```python
from build123d import *

# Parameters (mm, degrees)
F0_W     = 508
F0_H     = 457.2
F0_W_2   = 152.4
F0_H_2   = 101.6
F1_DEPTH = 12.7
F2_W     = 508
F2_H     = 228.6
F3_DEPTH = 12.701
F5_DEPTH = 12.701
F7_DEPTH = 9.525


with BuildPart() as f1:
    # F0 (on Top) → F1 (new body)
    with BuildSketch(Plane.XY):
        with Locations((76.2, -50.8)):
            Rectangle(F0_W, F0_H)
        with Locations((76.2, -50.8)):
            Rectangle(F0_W_2, F0_H_2, mode=Mode.SUBTRACT)
    extrude(amount=F1_DEPTH)

    # F2 (on face) → F3 (cut, through all)
    with BuildSketch(Plane.XY.offset(12.7)):
        with Locations((76.2, 63.5)):
            Rectangle(F2_W, F2_H)
    extrude(amount=-F3_DEPTH, mode=Mode.SUBTRACT)

    # F4 (on face) → F5 (cut, through all)
    with BuildSketch(Plane.XY.offset(12.7)):
        Polygon((-12.7, -63.5), (-165.1, -63.5), (-165.1, -266.7), (317.5, -266.7), (317.5, -63.5), (165.1, -63.5), (165.1, -114.3), (-12.7, -114.3), align=None)
    extrude(amount=-F5_DEPTH, mode=Mode.SUBTRACT)

    # F6 (on face) → F7 (cut)
    with BuildSketch(Plane(origin=(0, 0, 0), x_dir=(1, 0, 0), z_dir=(0, 0, -1))):
        Polygon((-174.625, 276.225), (-174.625, 53.975), (-3.175, 53.975), (-3.175, 104.775), (155.575, 104.775), (155.575, 53.975), (327.025, 53.975), (327.025, 276.225), align=None)
    extrude(amount=-F7_DEPTH, mode=Mode.SUBTRACT)


solid = f1.part
```
The listing builds one solid part. Answer for the finished solid, in the listing's coordinates (mm). A direction names the side the tool comes from. Coordinates: 2 decimals unless noted, no trailing zeros. Order: outer loops, then holes, each group sorted by start corner. A loop starts at its lowest first (then second) coordinate and runs counter-clockwise, first axis right, second up. Notation, with made-up numbers: M -20.5,45 L 9.5,45 A12 cw 9.5,56 Z; hole C 26,33.25 d4. An arc over 180 degrees is marked long. Answer as a JSON object with one key per item and string values. Group by question number.
1. Determine the mould class of faces 1 (the flat face through (240, -50.8, 6)), 2 (the flat face through (75, -101.6, 6)), 3 (the flat face through (-177.8, -167, 6)) for opening direction X: released by +X, released by -X, zero draft, split by the parting line, or undercut.
2. Section A-A on y = -121.5 is taken. Write down the section's boundary in (x, z) (3 decimals), then the cut area to 3 significant figures.
3. Straight lines are drawn through the part: line 1 (X direction, y = -107, z = 3.75) (3 decimals); line 2 (Y direction, x = -32, z = 5.75) (3 decimals); line 3 (X direction, y = -225, z = 11.5). For each, find the intervals that lie inside material, in ascending order.
4. Section C-C on z = 3 is taken. Write down the section's boundary in (x, y) (3 decimals).
5. A tool of negligible diameter and unlimited length cuts with its end or side. For faces 4 (the flat face through (-90, -50.8, 6)), 5 (the flat face through (-90, -53.975, 5)), 6 (the flat face through (152.4, -77, 6)), from which of +Z, -Z, +X, -X, +Y, -Y can it reach the whole face along a straight path? Write none if from no direction.
6. Section B-B on x = 136.5 is taken. Write down the section's boundary in (y, z) (3 decimals).
7. A flat-ended cylindrical pin translates along its axis: P1, Ø3, axis at x = 50, z = 8.5, coming from the +Y side. Find the tip coordinate at first contact, or state that the pin passes through.
Values follow:
{
 "1": {"face 1": "zero draft", "face 2": "undercut", "face 3": "released by -X"},
 "2": {"outline": "M -177.8,0 L -174.625,0 L -174.625,9.525 L -165.1,9.525 L -165.1,12.7 L -177.8,12.7 Z; M 317.5,9.525 L 327.025,9.525 L 327.025,0 L 330.2,0 L 330.2,12.7 L 317.5,12.7 Z", "area": "141 mm2"},
 "3": {"line 1": "-177.8 to -174.625, 327.025 to 330.2", "line 2": "-279.4 to -276.225, -53.975 to -50.8", "line 3": "-177.8 to -165.1, 317.5 to 330.2"},
 "4": {"outline": "M -177.8,-279.4 L 330.2,-279.4 L 330.2,-50.8 L 152.4,-50.8 L 152.4,-101.6 L 0,-101.6 L 0,-50.8 L -177.8,-50.8 Z; hole M -174.625,-276.225 L 327.025,-276.225 L 327.025,-53.975 L 155.575,-53.975 L 155.575,-104.775 L -3.175,-104.775 L -3.175,-53.975 L -174.625,-53.975 Z"},
 "5": {"face 4": "+Z, -Z, +X, -X, +Y", "face 5": "-Z", "face 6": "+Z, -Z, +Y"},
 "6": {"outline": "M -279.4,0 L -276.225,0 L -276.225,9.525 L -266.7,9.525 L -266.7,12.7 L -279.4,12.7 Z; M -114.3,9.525 L -104.775,9.525 L -104.775,0 L -101.6,0 L -101.6,12.7 L -114.3,12.7 Z"},
 "7": {"P1": "y = -101.6"}
}
